Check sheet for the modelled part. Datum: model origin and axes. Units: mm. A direction names the side the tool comes from. Coordinates: 2 decimals unless noted, no trailing zeros. Loops run counter-clockwise (first coordinate to the right, second up) from the corner with the lowest first, then second, coordinate; pieces in that order, holes last. Notation, with made-up numbers: M 44.5,80.25 L 69.5,80.25 A21 cw 69.5,108.25 Z; hole C 21.25,39 d4. An arc over 180 degrees is marked long. Return JSON: item names as keys, results as strings.
from build123d import *

# Parameters (mm, degrees)
SKETCH2_R             = 5.75
SKETCH2_R_2           = 4
BOSS_EXTRUDE1_DEPTH   = 12
BOSS_EXTRUDE2_DEPTH   = 6
M4X0_7_TAPPED_HOLE1_D = 3.3


with BuildPart() as part:
    # Sketch2 → Boss-Extrude1 (new body)
    with BuildSketch(Plane.XY):
        Circle(SKETCH2_R)
        Circle(SKETCH2_R_2, mode=Mode.SUBTRACT)
    extrude(amount=BOSS_EXTRUDE1_DEPTH)

    # Sketch3 → Boss-Extrude2 (add)
    with BuildSketch(Plane.XY):
        Polygon((-6.92820323, 0), (-3.464101615, 6), (3.464101615, 6), (6.92820323, 0), (3.464101615, -6), (-3.464101615, -6), align=None)
    extrude(amount=-BOSS_EXTRUDE2_DEPTH)

    # M4x0.7 Tapped Hole1 (through all)
    with Locations(Plane(origin=(0, 0, -6), x_dir=(-1, 0, 0), z_dir=(0, 0, -1))):
        with Locations((0, 0)):
            Hole(M4X0_7_TAPPED_HOLE1_D / 2)


solid = part.part
1) Go/stop test with flat-tipped pins: pin 1 Ø4.5 at (x, y) = (0, 0) entering from +Z; pin 2 Ø2 at (y, z) = (-2, 8.5) entering from +X; pin 3 Ø6 at (x, z) = (-3.5, 9.5) entering from -Y. Record where each tip stops, or that it passes through.
Answers:
{"pin 1": "z = 0", "pin 2": "x = 5.66", "pin 3": "y = -5.73"}
2) Scan lines: line 1 along Y through (x, z) = (0, -3.6); line 2 along Z through (x, y) = (3.25, 1); line 3 along Y through (x, z) = (-0.5, 9). Record each from-to range of solid material in increasing order. Write a range as [from, to].
Answers:
{"line 1": "[-6, -1.65], [1.65, 6]", "line 2": "[-6, 0]", "line 3": "[-5.73, -3.97], [3.97, 5.73]"}
3) Draft check along Y on faces 1 (the face through (0, 6, -3)), 2 (the face through (-2, 0, 0)), 3 (the face through (0, -6, -3)), 4 (the face through (-1.216, 1.115, -2.958)). Enter one of: +Y half, -Y half, draft (parallel to the pull), parting line (faces both ways), or undercut.
Answers:
{"face 1": "+Y half", "face 2": "undercut", "face 3": "-Y half", "face 4": "undercut"}
4) Section check C-C on y = 3.5. Record the cut outline in (x, z).
Answers:
{"outline": "M -4.91,-6 L 4.91,-6 L 4.91,0 L 4.56,0 L 4.56,12 L 1.94,12 L 1.94,0 L -1.94,0 L -1.94,12 L -4.56,12 L -4.56,0 L -4.91,0 Z"}
5) Section check D-D on x = -5.5. Record the cut outline in (y, z), then the cut area to 3 significant figures.
Answers:
{"outline": "M -2.47,-6 L 2.47,-6 L 2.47,0 L 1.68,0 L 1.68,12 L -1.68,12 L -1.68,0 L -2.47,0 Z", "area": "69.9 mm²"}
6) Set-up check for faces 5 (the face through (-0.867, -3.905, 5.916)), 6 (the face through (2, -4, 12)): record each of +Z, -Z, +X, -X, +Y, -Y from which the full face is reachable in a straight line by a thin tool's end or side.
Answers:
{"face 5": "+Z", "face 6": "+Z, +X, -X, +Y, -Y"}
7) Section check A-A on x = 0. Record the cut outline in (y, z).
Answers:
{"outline": "M -6,-6 L -1.65,-6 L -1.65,0 L -4,0 L -4,12 L -5.75,12 L -5.75,0 L -6,0 Z; M 1.65,-6 L 6,-6 L 6,0 L 5.75,0 L 5.75,12 L 4,12 L 4,0 L 1.65,0 Z"}
8) Section check B-B on z = -3. Record the cut outline in (x, y).
Answers:
{"outline": "M -6.93,0 L -3.46,-6 L 3.46,-6 L 6.93,0 L 3.46,6 L -3.46,6 Z; hole C 0,0 d3.3"}
